Build history of the part. All positions in model axes, mm. Face numbers are marked on the shaded views. A direction names the side the tool comes from. Give positions to 0.01 mm unless a question says otherwise; leave off trailing zeros. Loops run counter-clockwise (first coordinate to the right, second up) from the corner with the lowest first, then second, coordinate; pieces in that order, holes last.
1) Two-plate mould, pull along Y, no slides. Class the marked faces 1, 2 and 3: +Y half, -Y half, draft (parallel to the pull), parting line (faces both ways), or undercut.
2) Band-saw the part on B-B on z = 31. List the corners of the cut face in (x, y).
3) Flat gauge pins, fed straight in: P1, Ø10, axis at x = 3, z = 36, coming from the +Y side; P2, Ø8, axis at x = 35, y = -6, coming from the +Z side; P3, Ø10, axis at y = -6.5, z = 34, coming from the -X side. Where does each tip first touch, or does it go through?
4) Band-saw the part on A-A on x = 34. List the corners of the cut face in (y, z), then the cut area to 3 significant figures.
5) Wall check: line 1 (Y direction, x = 42, z = 3); line 2 (X direction, y = -21, z = 5); line 3 (X direction, y = -44.5, z = 16). Give the ranges that are in metal, low to high.
6) Band-saw the part on D-D on x = 27.5. List the corners of the cut face in (y, z), then the cut area to 3 significant figures.
7) 3-axis set-ups, long thin cutter, end or side, ignore diameter. For the marked faces 4, 5, 6 and 7: which of +Z, -Z, +X, -X, +Y, -Y reach the whole face in a straight line?
8) Band-saw the part on C-C on y = -44. List the corners of the cut face in (x, z), then the cut area to 3 significant figures.
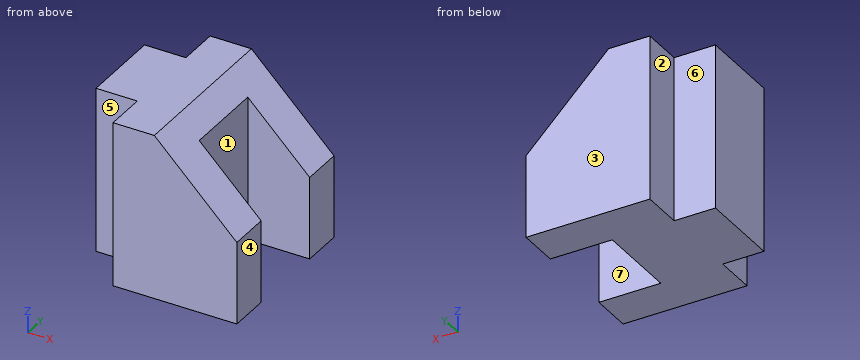
```python
from build123d import *

# Parameters (mm, degrees)
F0_W     = 50.8
F0_H     = 50.8
F1_DEPTH = 50.8
F3_DEPTH = 50.801
F4_W     = 12.7
F4_H     = 12.7030098811
F5_DEPTH = 50.801
F7_W     = 19.05
F7_H     = 25.4
F8_DEPTH = 76.201


with BuildPart() as f1:
    # F0 (on Front) → F1 (new body)
    with BuildSketch(Plane.XZ):
        with Locations((25.4, 25.4)):
            Rectangle(F0_W, F0_H)
    extrude(amount=F1_DEPTH)

    # F2 (on face) → F3 (cut, through all)
    with BuildSketch(Plane.XZ.offset(50.8)):
        Polygon((50.8, 50.8), (25.4, 50.8), (50.8, 25.4), align=None)
    extrude(amount=-F3_DEPTH, mode=Mode.SUBTRACT)

    # F4 (on face) → F5 (cut, through all)
    with BuildSketch(Plane.XY.offset(50.8)):
        with Locations((6.35, -6.3515049405)):
            Rectangle(F4_W, F4_H)
        with Locations((6.35, -44.4484950595)):
            Rectangle(F4_W, F4_H)
    extrude(amount=-F5_DEPTH, mode=Mode.SUBTRACT)

    # F7 (on offset) → F8 (cut, through all)
    with BuildSketch(Plane.XY.offset(76.2)):
        with Locations((41.275, -25.4)):
            Rectangle(F7_W, F7_H)
    extrude(amount=-F8_DEPTH, mode=Mode.SUBTRACT)


solid = f1.part
```
Findings below:
1. face 1: undercut
1. face 2: draft
1. face 3: +Y half
2. outline: (0, -38.1) - (12.7, -38.1) - (12.7, -50.8) - (45.2, -50.8) - (45.2, -38.1) - (31.75, -38.1) - (31.75, -12.7) - (45.2, -12.7) - (45.2, 0) - (12.7, 0) - (12.7, -12.7) - (0, -12.7) - close
3. P1: stops at y = -12.7
3. P2: stops at z = 45.2
3. P3: stops at x = 12.7
4. outline: (-50.8, 0) - (-38.1, 0) - (-38.1, 42.2) - (-50.8, 42.2) - close; (-12.7, 0) - (0, 0) - (0, 42.2) - (-12.7, 42.2) - close
4. area: 1,070 mm2
5. line 1: y = -50.8 to -38.1, -12.7 to 0
5. line 2: x = 0 to 31.75
5. line 3: x = 12.7 to 50.8
6. outline: (-50.8, 0) - (0, 0) - (0, 48.7) - (-50.8, 48.7) - close
6. area: 2,470 mm2
7. face 4: +Z, -Z, +X, +Y, -Y
7. face 5: +Z, -Z, -X, -Y
7. face 6: +Z, -Z, -X, +Y
7. face 7: +Z, -Z, +X
8. outline: (12.7, 0) - (50.8, 0) - (50.8, 25.4) - (25.4, 50.8) - (12.7, 50.8) - close
8. area: 1,610 mm2
